The figure shows three views and two pictorial views of one solid part (mm, origin at its lowest corner). Answer the questions. A direction names the side the tool comes from. Coordinates: 2 decimals unless noted, no trailing zeros. Write each loop counter-clockwise with the first axis right and the second up, starting at its lowest first coordinate (ties: lowest second). Pieces come first, ordered by that corner, then holes.
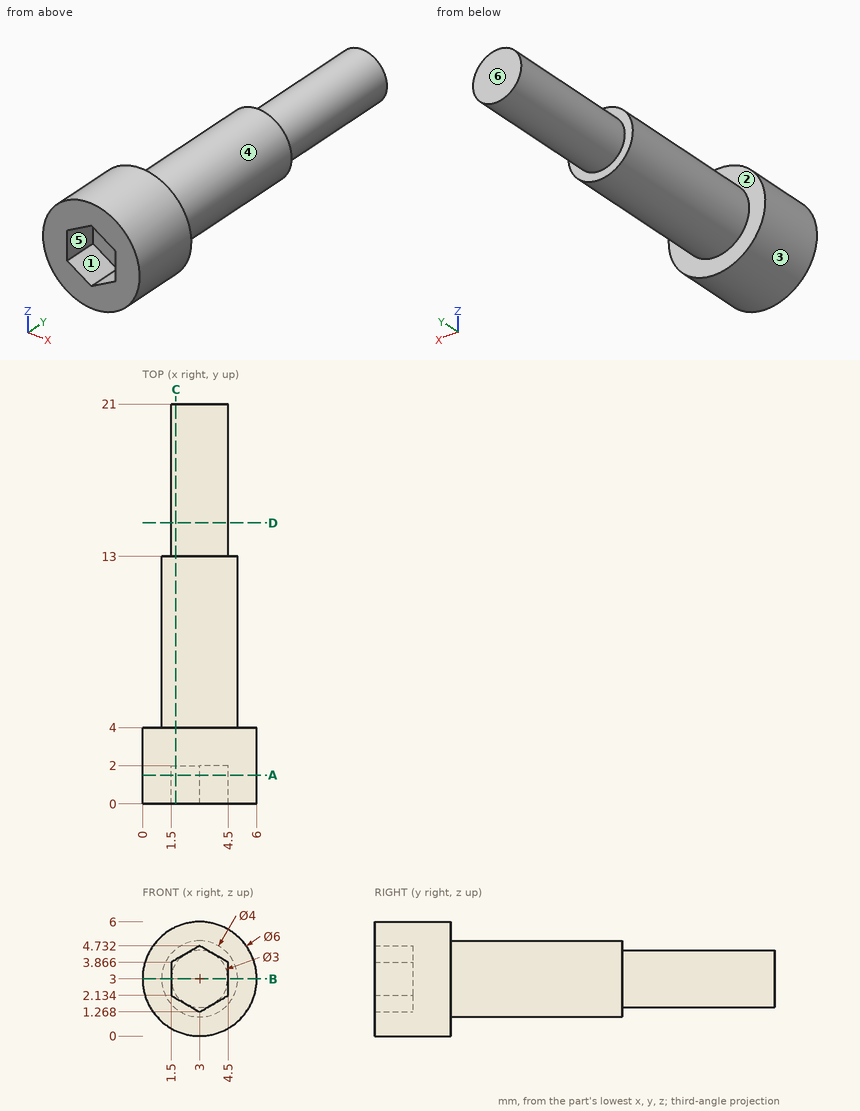
1. Section D-D on y = 14.75 is taken. Give the vertices of the cut face in (x, z).
Results found:
outline: circle Ø3 at (3, 3)
2. Flat-ended cylindrical pins translate along their axes: P1, Ø1.5, axis at x = 2.5, z = 3, coming from the -Y side; P2, Ø1, axis at y = 12.5, z = 3.5, coming from the +X side; P3, Ø0.5, axis at y = 1, z = 3.5, coming from the -X side. Find the tip coordinate at first contact, or state that the pin passes through.
Results found:
P1: stops at y = 2
P2: stops at x = 5
P3: stops at x = 0.01
3. Section A-A on y = 1.5 is taken. Give the vertices of the cut face in (x, z).
Results found:
outline: circle Ø6 at (3, 3); hole (1.5, 2.13) - (3, 1.27) - (4.5, 2.13) - (4.5, 3.87) - (3, 4.73) - (1.5, 3.87) - close
4. Find the intervals of material crossed by L1, parallel to Y at x = 5.15, z = 4.95; L2, parallel to Y at x = 1.8, z = 4.4; L3, parallel to Z at x = 2.95, y = 12.5, in increasing order.
Results found:
L1: y = 0 to 4
L2: y = 0 to 13
L3: z = 1 to 5
5. For a pull along Z with two mould halves and no side action, classify the marked faces 1, 2 and 3 as pulls with the +Z half, pulls with the -Z half, needs draft (parallel to the pull), parting line crosses it, or undercut.
Results found:
face 1: undercut
face 2: needs draft
face 3: parting line crosses it
6. Section B-B on z = 3 is taken. Give the vertices of the cut face in (x, y), then the cut area to 3 significant figures.
Results found:
outline: (0, 0) - (1.5, 0) - (1.5, 2) - (4.5, 2) - (4.5, 0) - (6, 0) - (6, 4) - (5, 4) - (5, 13) - (4.5, 13) - (4.5, 21) - (1.5, 21) - (1.5, 13) - (1, 13) - (1, 4) - (0, 4) - close
area: 78.0 mm2
7. A tool of negligible diameter and unlimited length cuts with its end or side. For the marked faces 4, 5 and 6, from which of +Z, -Z, +X, -X, +Y, -Y can it reach the whole face along a straight path? Write none if from no direction.
Results found:
face 4: +Y
face 5: -Y
face 6: +Z, -Z, +X, -X, +Y
8. Section C-C on x = 1.75 is taken. Give the vertices of the cut face in (y, z).
Results found:
outline: (0, 0.27) - (4, 0.27) - (4, 1.44) - (13, 1.44) - (13, 2.17) - (21, 2.17) - (21, 3.83) - (13, 3.83) - (13, 4.56) - (4, 4.56) - (4, 5.73) - (0, 5.73) - (0, 4.01) - (2, 4.01) - (2, 1.99) - (0, 1.99) - close
